```python
from build123d import *

# Parameters (mm, degrees)
SKETCH2_R                = 48.5
BOSS_EXTRUDE1_DEPTH      = 4
SKETCH4_R                = 1.5
CUT_EXTRUDE2_DEPTH       = 5
SKETCH5_R                = 3.75
CUT_EXTRUDE3_DEPTH       = 1.5
BOSS_EXTRUDE2_DEPTH      = 14
CUT_EXTRUDE5_REACH       = 44.5
SKETCH9_R                = 1.3
CUT_EXTRUDE6_DEPTH       = 67.5
CUT_EXTRUDE9_REACH       = 46.5
SKETCH11_R               = 9
BOSS_EXTRUDE7_DEPTH      = 9
BOSS_EXTRUDE7_DEPTH_BACK = 14
BOSS_EXTRUDE10_DEPTH     = 9
SKETCH27_W               = 16
SKETCH27_H               = 6
BOSS_EXTRUDE11_DEPTH     = 12
FILLET6_R                = 3
CUT_EXTRUDE16_REACH      = 77.672
SKETCH28_W               = 8
SKETCH28_H               = 4
CUT_EXTRUDE17_DEPTH      = 49.5
CUT_EXTRUDE17_DEPTH_BACK = 57.89561214


with BuildPart() as part:
    # Sketch2 → Boss-Extrude1 (new body)
    with BuildSketch(Plane(origin=(0, 0, 0), x_dir=(1, 0, 0), z_dir=(0, 1, 0))):
        Circle(SKETCH2_R)
    extrude(amount=BOSS_EXTRUDE1_DEPTH)

    # Sketch4 → Cut-Extrude2 (cut, through all)
    with BuildSketch(Plane.XZ):
        with Locations((0, 7.25)):
            Circle(SKETCH4_R)
        with Locations((0, -7.25)):
            Circle(SKETCH4_R)
    extrude(amount=-CUT_EXTRUDE2_DEPTH, mode=Mode.SUBTRACT)

    # Sketch5 → Cut-Extrude3 (cut)
    with BuildSketch(Plane.XZ):
        Circle(SKETCH5_R)
    extrude(amount=-CUT_EXTRUDE3_DEPTH, mode=Mode.SUBTRACT)

    # Sketch7 → Boss-Extrude2 (add)
    with BuildSketch(Plane(origin=(-4, 0, 0), x_dir=(0, 0, -1), z_dir=(1, 0, 0))):
        with BuildLine():
            Line((35.838240239, 4), (35.838240239, 24.116109522))
            ThreePointArc((35.838240239, 24.116109522), (38.028688753, 32.721810064), (44.066915997, 39.233027943))
            ThreePointArc((44.066915997, 39.233027943), (49.118651286, 70.801932352), (17.192816244, 72.492142963))
            Line((17.192816244, 72.492142963), (-21.454056035, 33.845270684))
            ThreePointArc((-21.454056035, 33.845270684), (-26.873374818, 25.734686963), (-28.776386505, 16.167601154))
            Line((-28.776386505, 16.167601154), (-28.776386505, 4))
            Line((-28.776386505, 4), (35.838240239, 4))
        make_face()
    extrude(amount=-BOSS_EXTRUDE2_DEPTH)

    # Sketch8 → Cut-Extrude5 (cut, up to next)
    with BuildSketch(Plane(origin=(-6, 0, 0), x_dir=(0, 0, -1), z_dir=(1, 0, 0)), mode=Mode.PRIVATE) as cut_extrude5_sk1:
        Polygon((3.227457316, 42.970434849), (32.218835345, 71.961812877), (47.06807775, 57.112570472), (18.076699721, 28.121192444), align=None)
    cut_extrude5_tool1 = extrude(cut_extrude5_sk1.sketch, amount=-CUT_EXTRUDE5_REACH, mode=Mode.PRIVATE) & part.part
    add(cut_extrude5_tool1.solids().sort_by_distance((-6, 50.041503, -25.147768))[0], mode=Mode.SUBTRACT)

    # Sketch9 → Cut-Extrude6 (cut, through all)
    with BuildSketch(Plane.ZY.offset(18)):
        with Locations((-38.582796375, 70.547599315)):
            Circle(SKETCH9_R)
        with Locations((-45.653864187, 63.476531503)):
            Circle(SKETCH9_R)
        with Locations((-11.71273869, 29.535406006)):
            Circle(SKETCH9_R)
        with Locations((-4.641670878, 36.606473818)):
            Circle(SKETCH9_R)
    extrude(amount=-CUT_EXTRUDE6_DEPTH, mode=Mode.SUBTRACT)

    # Sketch11 → Cut-Extrude9 (cut, up to next)
    with BuildSketch(Plane(origin=(-4, 0, 0), x_dir=(0, 0, -1), z_dir=(1, 0, 0)), mode=Mode.PRIVATE) as cut_extrude9_sk1:
        with Locations((32.39561204, 57.289347168)):
            Circle(SKETCH11_R)
    cut_extrude9_tool1 = extrude(cut_extrude9_sk1.sketch, amount=-CUT_EXTRUDE9_REACH, mode=Mode.PRIVATE) & part.part
    add(cut_extrude9_tool1.solids().sort_by_distance((-4, 57.289347, -32.395612))[0], mode=Mode.SUBTRACT)

    # Sketch17 → Boss-Extrude7 (add, two sides)
    with BuildSketch(Plane.ZY.offset(18)) as boss_extrude7_sk:
        with BuildLine():
            ThreePointArc((28.776386505, 16.167601154), (27.123973821, 25.105731079), (22.385173182, 32.862302662))
            ThreePointArc((22.385173182, 32.862302662), (21.926270321, 33.360091302), (21.454056035, 33.845270684))
            Line((21.454056035, 33.845270684), (-17.192816244, 72.492142963))
            Line((-17.192816244, 72.492142963), (20.153274432, 30.85765023))
            ThreePointArc((20.153274432, 30.85765023), (24.322572701, 24.032347355), (25.776386505, 16.167601154))
            Line((25.776386505, 16.167601154), (25.776386505, 4))
            Line((25.776386505, 4), (28.776386505, 4))
            Line((28.776386505, 4), (28.776386505, 16.167601154))
        make_face()
        with BuildLine():
            Line((22.385173182, 32.862302662), (-15.071495901, 74.613463307))
            ThreePointArc((-15.071495901, 74.613463307), (-51.452098623, 72.687409354), (-45.695470037, 36.713541539))
            ThreePointArc((-45.695470037, 36.713541539), (-40.663614001, 31.28752664), (-38.838240239, 24.116109522))
            Line((-38.838240239, 24.116109522), (-38.838240239, 4))
            Line((-38.838240239, 4), (-35.838240239, 4))
            Line((-35.838240239, 4), (-35.838240239, 24.116109522))
            ThreePointArc((-35.838240239, 24.116109522), (-38.028688753, 32.721810064), (-44.066915997, 39.233027943))
            ThreePointArc((-44.066915997, 39.233027943), (-49.118651286, 70.801932352), (-17.192816244, 72.492142963))
            Line((-17.192816244, 72.492142963), (21.454056035, 33.845270684))
            ThreePointArc((21.454056035, 33.845270684), (21.926270321, 33.360091302), (22.385173182, 32.862302662))
        make_face()
    extrude(amount=BOSS_EXTRUDE7_DEPTH)
    extrude(boss_extrude7_sk.sketch, amount=-BOSS_EXTRUDE7_DEPTH_BACK)

    # Sketch25 → Boss-Extrude10 (add)
    with BuildSketch(Plane.ZY.offset(18)):
        with BuildLine():
            ThreePointArc((-44.066915997, 39.233027943), (-38.028688753, 32.721810064), (-35.838240239, 24.116109522))
            Line((-35.838240239, 24.116109522), (-35.838240239, 4))
            Line((-35.838240239, 4), (-27.838240239, 4))
            add(Edge.make_bspline(
                [(-44.066915997, 39.233027943), (-36.217415427, 34.159241535), (-9.669096592, 17.105596636), (-27.838240239, 4)],
                knots=[0, 0, 0, 0, 1, 1, 1, 1], degree=3))
        make_face()
        with BuildLine():
            add(Edge.make_bspline(
                [(10.649740153, 41.452462744), (25.981861033, 24.35977476), (19.776386505, 4)],
                knots=[0, 0, 0, 1, 1, 1], degree=2))
            Line((19.776386505, 4), (25.776386505, 4))
            Line((25.776386505, 4), (25.776386505, 16.167601154))
            ThreePointArc((25.776386505, 16.167601154), (24.322572701, 24.032347355), (20.153274432, 30.85765023))
            Line((20.153274432, 30.85765023), (10.649740153, 41.452462744))
        make_face()
    extrude(amount=BOSS_EXTRUDE10_DEPTH)

    # Sketch27 → Boss-Extrude11 (add)
    with BuildSketch(Plane(origin=(0, 4, 0), x_dir=(1, 0, 0), z_dir=(0, 1, 0))):
        with Locations((6, -15.776386505)):
            Rectangle(SKETCH27_W, SKETCH27_H)
    extrude(amount=BOSS_EXTRUDE11_DEPTH)

    # Fillet6
    fillet6_edges = [part.edges().sort_by_distance(p)[0] for p in [
        (-2, 16, 15.776386505),
        (14, 16, 15.776386505),
    ]]
    fillet(fillet6_edges, radius=FILLET6_R)

    # Sketch28 → Cut-Extrude16 (cut, up to next)
    with BuildSketch(Plane.XY.offset(18.776386505), mode=Mode.PRIVATE) as cut_extrude16_sk1:
        with Locations((6, 10)):
            Rectangle(SKETCH28_W, SKETCH28_H)
    cut_extrude16_tool1 = extrude(cut_extrude16_sk1.sketch, amount=-CUT_EXTRUDE16_REACH, mode=Mode.PRIVATE) & part.part
    add(cut_extrude16_tool1.solids().sort_by_distance((6, 10, 18.776387))[0], mode=Mode.SUBTRACT)

    # Sketch29 → Cut-Extrude17 (cut, two sides)
    with BuildSketch(Plane.XY) as cut_extrude17_sk:
        with BuildLine():
            Line((-21, 81.789347168), (-27, 81.789347168))
            Line((-27, 81.789347168), (-27, 4))
            Line((-27, 4), (-26.5, 4))
            add(Edge.make_bspline(
                [(-21, 81.789347168), (-19.81566604, 42.545643995), (-26.5, 4)],
                knots=[0, 0, 0, 1, 1, 1], degree=2))
        make_face()
    extrude(amount=CUT_EXTRUDE17_DEPTH, mode=Mode.SUBTRACT)
    extrude(cut_extrude17_sk.sketch, amount=-CUT_EXTRUDE17_DEPTH_BACK, mode=Mode.SUBTRACT)


solid = part.part
```
Design review of the part built by this model. Coordinates are the model's own, in mm. A direction names the side the tool comes from. Give positions to 0.01 mm unless a question says otherwise; leave off trailing zeros. Loops run counter-clockwise (first coordinate to the right, second up) from the corner with the lowest first, then second, coordinate; pieces in that order, holes last. Notation, with made-up numbers: (-19, 81) -> (-1, 81) arc R26 ccw to (-1, 101) -> close; hole circle Ø2 at (-12, 82.25). An arc over 180 degrees is marked (long way). Write each question's results on one line, items separated by ' | '.
Q1. The part is to be moulded in two halves that separate along Z. For faces 6 (the face through (-15, 10, 28.776)), 7 (the face through (-15, 14, -38.838)), 8 (the face through (-11.098, 28.266, -11.995)), say which applies: +Z half, -Z half, draft (parallel to the pull), parting line (faces both ways), or undercut.
Reply:
face 6: +Z half | face 7: -Z half | face 8: undercut
Q2. Take a section at B-B, the plane x = -40. Write out the cut boundary in (y, z), plus the area to 3 significant figures.
Reply:
outline: (0, -27.43) -> (4, -27.43) -> (4, 27.43) -> (0, 27.43) -> close | area: 219 mm²
Q3. For pin 1 Ø10 at (y, z) = (54, -23) entering from -X; pin 2 Ø3.5 at (y, z) = (29.54, -11.71) entering from +X; pin 3 Ø3 at (y, z) = (9, 15.5) entering from +X, all flat-tipped, find the tip position at first contact; note any pin that passes through.
Reply:
pin 1: stops at x = -6 | pin 2: stops at x = -4 | pin 3: stops at x = 14
Q4. Wall thickness on L1, parallel to Z at x = 0, y = 1; L2, parallel to Z at x = 0, y = 2.6; L3, parallel to Z at x = -21, y = 14.5: over which ranges is each line inside the solid? List them lowest first.
Reply:
L1: z = -48.5 to -8.75, -5.75 to -3.75, 3.75 to 5.75, 8.75 to 48.5 | L2: z = -48.5 to -8.75, -5.75 to 5.75, 8.75 to 48.5 | L3: z = -38.84 to -21.61, 21.55 to 28.78
Q5. Take a section at A-A, the plane x = 17.5. Write out the cut boundary in (y, z), plus the area to 3 significant figures.
Reply:
outline: (0, -45.23) -> (4, -45.23) -> (4, 45.23) -> (0, 45.23) -> close | area: 362 mm²
Q6. Machinability: for faces 1 (the face through (-3.746, 0.74, 0.165)), 2 (the face through (-2, 8, 16)), 3 (the face through (6, 12, 16)), 4 (the face through (-11.916, 42.82, -32.775)), 5 (the face through (6, 7, 18.776)), which of the approach directions +Z, -Z, +X, -X, +Y, -Y give a long, thin tool a straight path to every point of the face, cutting with its end or side? Answer none if there is none.
Reply:
face 1: -Y | face 2: +Z, -Z, +Y | face 3: +Z, -Z | face 4: -X | face 5: +Z, +X, +Y
